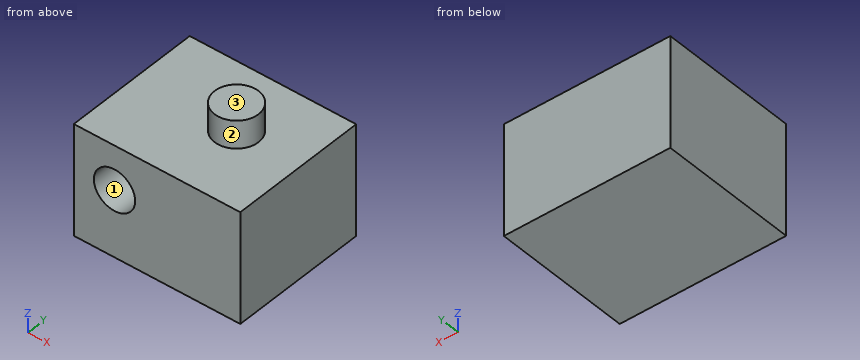
```python
from build123d import *

# Parameters (mm, degrees)
F0_W     = 38.1
F0_H     = 31.75
F1_DEPTH = 25.4
F2_R     = 4.729521
F3_DEPTH = 25.4
F4_R     = 5.03132
F5_DEPTH = 6.35


with BuildPart() as f1:
    # F0 (on Top) → F1 (new body)
    with BuildSketch(Plane.XY):
        with Locations((19.05, 15.875)):
            Rectangle(F0_W, F0_H)
    extrude(amount=F1_DEPTH)

    # F2 (on Front) → F3 (cut)
    with BuildSketch(Plane.XZ):
        with Locations((9.311019, 15.262362)):
            Circle(F2_R)
    extrude(amount=-F3_DEPTH, mode=Mode.SUBTRACT)

    # F4 (on face) → F5 (join)
    with BuildSketch(Plane.XY.offset(25.4)):
        with Locations((23.096351, 16.941737)):
            Circle(F4_R)
    extrude(amount=F5_DEPTH)


solid = f1.part
```
Model file for the job. Use its own axes, mm. Face numbers are marked on the shaded views. Round coordinates to 2 decimals unless told otherwise and drop trailing zeros. Order: outer loops, then holes, each group sorted by start corner. A loop starts at its lowest first (then second) coordinate and runs counter-clockwise, first axis right, second up. Notation, with made-up numbers: M 70,12 L 86,12 A26 ccw 86,48 Z; hole C 24,25.5 d4. An arc over 180 degrees is marked long. Use CSV: the item, a comma, the result in double quotes.
Item 1: Pull direction Z, two halves, no side cores. Call the marked faces 1, 2 and 3: released by +Z, released by -Z, zero draft, split by the parting line, or undercut.
Worked answers:
face 1,"undercut"
face 2,"zero draft"
face 3,"released by +Z"
Item 2: Saw through at D-D (y = 27.5). List the corners of the cut face in (x, z).
Worked answers:
outline,"M 0,0 L 38.1,0 L 38.1,25.4 L 0,25.4 Z"
Item 3: Saw through at C-C (y = 20). List the corners of the cut face in (x, z), plus the area to 3 significant figures.
Worked answers:
outline,"M 0,0 L 38.1,0 L 38.1,25.4 L 27.09,25.4 L 27.09,31.75 L 19.1,31.75 L 19.1,25.4 L 0,25.4 Z; hole C 9.31,15.26 d9.46"
area,"948 mm²"
Item 4: Saw through at B-B (x = 7.5). List the corners of the cut face in (y, z), plus the area to 3 significant figures.
Worked answers:
outline,"M 0,0 L 31.75,0 L 31.75,25.4 L 0,25.4 L 0,19.63 L 25.4,19.63 L 25.4,10.89 L 0,10.89 Z"
area,"585 mm²"
Item 5: Probe probe 1 along Z at (x, y) = (28.5, 17); probe 2 along Y at (x, z) = (9.5, 13); probe 3 along Z at (x, y) = (11, 7). List the from-to ranges inside material, lowest first.
Worked answers:
probe 1,"0 to 25.4"
probe 2,"25.4 to 31.75"
probe 3,"0 to 10.84, 19.68 to 25.4"
Item 6: Pin check, flat tips, straight feed: pin 1 (8 mm diameter, centred on y = 20.5, z = 15, fed in from -X); pin 2 (1.5 mm diameter, centred on x = 33, y = 21.5, fed in from +Z). Stop position of each tip, or through.
Worked answers:
pin 1,"x = 0"
pin 2,"z = 25.4"
Item 7: Saw through at A-A (z = 13.5). List the corners of the cut face in (x, y).
Worked answers:
outline,"M 0,0 L 4.92,0 L 4.92,25.4 L 13.7,25.4 L 13.7,0 L 38.1,0 L 38.1,31.75 L 0,31.75 Z"
